Geometry check sheet. Reference: the model listing, model coordinates, mm. Face numbers are marked on the shaded views. Round coordinates to 2 decimals unless told otherwise and drop trailing zeros. Order: outer loops, then holes, each group sorted by start corner. A loop starts at its lowest first (then second) coordinate and runs counter-clockwise, first axis right, second up. Notation, with made-up numbers: (-27, 59) -> (17, 59) arc R20 ccw to (17, 70) -> close; hole circle Ø10 at (70, -17). An arc over 180 degrees is marked (long way). Use a Markdown table: item, result. Add a question column.
Item 1: Sectioned sample at A-A, the plane x = 35. Record the cut outline in (y, z).
Item 2: Material ranges on probe 1 along Z at (x, y) = (-0.5, -6.75); probe 2 along X at (y, z) = (-8, -2); probe 3 along Z at (x, y) = (-37, -2), recorded low to high. Write a range as [from, to].
Item 3: Sectioned sample at D-D, the plane x = -44. Record the cut outline in (y, z), and give its area (3 significant figures).
Item 4: Sectioned sample at C-C, the plane y = -5.25. Record the cut outline in (x, z), and give its area (3 significant figures).
Item 5: Mould release check, pull along X, two halves, no side actions. Record for the marked faces 1, 2, 3 and 4: pulls with the +X half, pulls with the -X half, needs draft (parallel to the pull), parting line crosses it, or undercut.
Item 6: Gauge pin test, flat ends, axial feed: pin 1 Ø6 at (x, y) = (-6.5, -5) entering from +Z; pin 2 Ø5 at (x, z) = (-19, 4) entering from -Y; pin 3 Ø5 at (x, y) = (37.5, -3) entering from -Z; pin 4 Ø9.5 at (x, z) = (35, 0) entering from -Y. Record the tip position at first contact, or that the pin passes through.
Item 7: Sectioned sample at B-B, the plane z = 10. Record the cut outline in (x, y).
from build123d import *

# Parameters (mm, degrees)
F0_R     = 6
F1_DEPTH = 10


with BuildPart() as f1:
    # F0 (on Front) → F1 (new body)
    with BuildSketch(Plane.XZ):
        with BuildLine():
            Line((41.428571, 13.552619), (12.857143, 27.105237))
            ThreePointArc((12.857143, 27.105237), (6.589495, 29.267363), (0, 30))
            ThreePointArc((0, 30), (-6.589495, 29.267363), (-12.857143, 27.105237))
            Line((-12.857143, 27.105237), (-41.428571, 13.552619))
            ThreePointArc((-41.428571, 13.552619), (-47.677314, 8.017837), (-50, 0))
            ThreePointArc((-50, 0), (-47.677314, -8.017837), (-41.428571, -13.552619))
            Line((-41.428571, -13.552619), (-12.857143, -27.105237))
            ThreePointArc((-12.857143, -27.105237), (-6.589495, -29.267363), (0, -30))
            ThreePointArc((0, -30), (6.589495, -29.267363), (12.857143, -27.105237))
            Line((12.857143, -27.105237), (41.428571, -13.552619))
            ThreePointArc((41.428571, -13.552619), (47.677314, -8.017837), (50, 0))
            ThreePointArc((50, 0), (47.677314, 8.017837), (41.428571, 13.552619))
        make_face()
        with Locations((-35, 0)):
            Circle(F0_R, mode=Mode.SUBTRACT)
        with BuildLine():
            ThreePointArc((0, 21), (14.849242, 14.849242), (21, 0))
            ThreePointArc((21, 0), (14.849242, -14.849242), (0, -21))
            ThreePointArc((0, -21), (-14.849242, -14.849242), (-21, 0))
            ThreePointArc((-21, 0), (-14.849242, 14.849242), (0, 21))
        make_face(mode=Mode.SUBTRACT)
        with Locations((35, 0)):
            Circle(F0_R, mode=Mode.SUBTRACT)
    extrude(amount=F1_DEPTH)


solid = f1.part
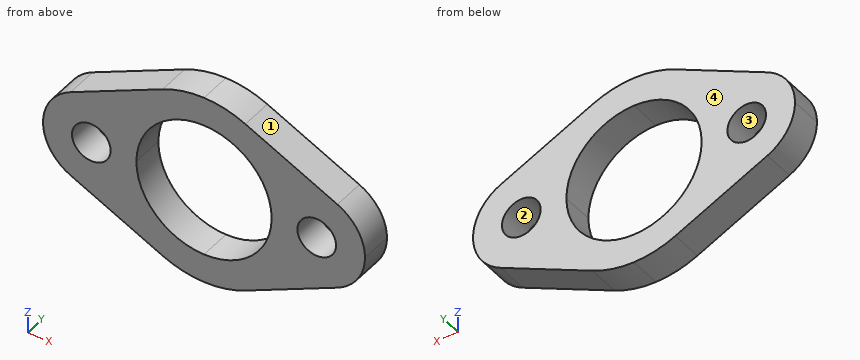
Found:
| question | item | result |
|---|---|---|
| 1 | outline | (-10, -16.6) -> (0, -16.6) -> (0, -6) -> (-10, -6) -> close; (-10, 6) -> (0, 6) -> (0, 16.6) -> (-10, 16.6) -> close |
| 2 | probe 1 | z = [-30, -20.99], [20.99, 30] |
| 2 | probe 2 | x = [-49.87, -40.66], [-29.34, -20.9], [20.9, 29.34], [40.66, 49.87] |
| 2 | probe 3 | z = [-15.65, -5.66], [5.66, 15.65] |
| 3 | outline | (-10, -12) -> (0, -12) -> (0, 12) -> (-10, 12) -> close |
| 3 | area | 240 mm2 |
| 4 | outline | (-41.43, -13.55) -> (-12.86, -27.11) arc R30 ccw to (0, -30) arc R30 ccw to (12.86, -27.11) -> (41.43, -13.55) arc R15 ccw to (41.43, 13.55) -> (12.86, 27.11) arc R30 ccw to (0, 30) arc R30 ccw to (-12.86, 27.11) -> (-41.43, 13.55) arc R15 ccw to start; hole circle Ø12 at (-35, 0); hole (-21, 0) arc R21 ccw to (0, -21) arc R21 ccw to (21, 0) arc R21 ccw to (0, 21) arc R21 ccw to start; hole circle Ø12 at (35, 0) |
| 4 | area | 2,540 mm2 |
| 5 | face 1 | pulls with the +X half |
| 5 | face 2 | undercut |
| 5 | face 3 | undercut |
| 5 | face 4 | needs draft |
| 6 | pin 1 | stops at z = 29.8 |
| 6 | pin 2 | stops at y = -10 |
| 6 | pin 3 | stops at z = -16.6 |
| 6 | pin 4 | passes through |
| 7 | outline | (-46.18, -10) -> (-18.47, -10) -> (-18.47, 0) -> (-46.18, 0) -> close; (18.47, -10) -> (46.18, -10) -> (46.18, 0) -> (18.47, 0) -> close |
